from build123d import *

# Parameters (mm, degrees)
ESQUISSE1_W        = 140
ESQUISSE1_H        = 50
ESQUISSE1_R        = 4.05
ESQUISSE1_R_2      = 1.55
ESQUISSE1_W_2      = 12
ESQUISSE1_H_2      = 4
BOSS_EXTRU_1_DEPTH = 5


with BuildPart() as part:
    # Esquisse1 → Boss.-Extru.1 (new body)
    with BuildSketch(Plane.XY):
        Rectangle(ESQUISSE1_W, ESQUISSE1_H)
        with Locations((-40, 0)):
            Circle(ESQUISSE1_R, mode=Mode.SUBTRACT)
        with Locations((-55, -13)):
            Circle(ESQUISSE1_R_2, mode=Mode.SUBTRACT)
        with Locations(Location((-55, 13, 0), (0, 0, 180))):
            Circle(ESQUISSE1_R_2, mode=Mode.SUBTRACT)
        with Locations(Location((55, -13, 0), (0, 0, 180))):
            Circle(ESQUISSE1_R_2, mode=Mode.SUBTRACT)
        with Locations((55, 13)):
            Circle(ESQUISSE1_R_2, mode=Mode.SUBTRACT)
        with Locations(Location((40, 0, 0), (0, 0, 180))):
            Circle(ESQUISSE1_R, mode=Mode.SUBTRACT)
        with Locations((-12, 12)):
            Circle(ESQUISSE1_R_2, mode=Mode.SUBTRACT)
        with Locations(Location((-12, -12, 0), (0, 0, 180))):
            Circle(ESQUISSE1_R_2, mode=Mode.SUBTRACT)
        with Locations((12, -12)):
            Circle(ESQUISSE1_R_2, mode=Mode.SUBTRACT)
        with Locations(Location((12, 12, 0), (0, 0, 180))):
            Circle(ESQUISSE1_R_2, mode=Mode.SUBTRACT)
        with Locations((0, 12)):
            Rectangle(ESQUISSE1_W_2, ESQUISSE1_H_2, mode=Mode.SUBTRACT)
    extrude(amount=-BOSS_EXTRU_1_DEPTH)


solid = part.part
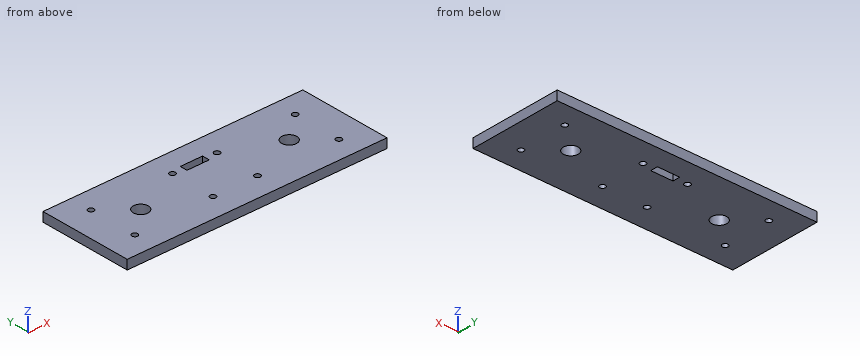
Design review of the part built by this model. Coordinates are the model's own, in mm. Round coordinates to 2 decimals unless told otherwise and drop trailing zeros. Loops run counter-clockwise (first coordinate to the right, second up) from the corner with the lowest first, then second, coordinate; pieces in that order, holes last. Notation, with made-up numbers: M -31,18.5 L 25,18.5 A25 cw 25,30.5 Z; hole C 57,38.25 d6. An arc over 180 degrees is marked long. Answer as a JSON object with one key per item and string values.
Item 1: Wall thickness on L1, parallel to Y at x = -12, z = -1.15; L2, parallel to Y at x = -55, z = -3.2; L3, parallel to Y at x = 0, z = -1.8: over which ranges is each line inside the solid? List them lowest first. Write a range as from..to.
Answer sheet:
{"L1": "y = -25..-13.55, -10.45..10.45, 13.55..25", "L2": "y = -25..-14.55, -11.45..11.45, 14.55..25", "L3": "y = -25..10, 14..25"}
Item 2: We need section A-A on x = 55. Give the boundary of the cut face in (y, z), and give its area (3 significant figures).
Answer sheet:
{"outline": "M -25,-5 L -14.55,-5 L -14.55,0 L -25,0 Z; M -11.45,-5 L 11.45,-5 L 11.45,0 L -11.45,0 Z; M 14.55,-5 L 25,-5 L 25,0 L 14.55,0 Z", "area": "219 mm^2"}
Item 3: We need section C-C on z = -3.4. State how many separate pieces and enclosed holes the cut face has, and give its area (3 significant figures).
Answer sheet:
{"separate pieces": "1", "enclosed holes": "11", "area": "6,790 mm^2"}
Item 4: We need section B-B on y = 0. Give the boundary of the cut face in (x, z).
Answer sheet:
{"outline": "M -70,-5 L -44.05,-5 L -44.05,0 L -70,0 Z; M -35.95,-5 L 35.95,-5 L 35.95,0 L -35.95,0 Z; M 44.05,-5 L 70,-5 L 70,0 L 44.05,0 Z"}
